Geometry: final body of the model. Coordinates: model frame, mm. A direction names the side the tool comes from. Give positions to 0.01 mm unless a question says otherwise; leave off trailing zeros. Write each loop counter-clockwise with the first axis right and the second up, starting at its lowest first coordinate (ties: lowest second). Pieces come first, ordered by that corner, then holes.
Q1. Mould query, pull axis X, two halves, no side actions, for faces 3 (the cylindrical face through (19.14, -19.1, 0.28)), 4 (the cylindrical face through (-19.1, -19.14, 0.28)), 5 (the cylindrical face through (-17, -16.5, 0)), 6 (the cylindrical face through (12.5, 15.1, 0)). Classes: +X half, -X half, draft (parallel to the pull), parting line (faces both ways), or undercut.
Q2. Line query: line 1 (Y direction, x = -15, z = 1.2); line 2 (Y direction, x = 13, z = 0); line 3 (Z direction, x = 12.5, y = -12). Output: solid intervals per line, ascending.
Q3. Section D-D (y = 0). Return the cut outline in (x, z).
Q4. Section A-A (z = 1.5). Return the cut outline in (x, y), plus the area to 3 significant figures.
Q5. Section B-B (x = 15). Return the cut outline in (y, z), plus the area to 3 significant figures.
Q6. Pin query (flat end, axial travel): pin 1 Ø6.5 at (x, y) = (-15, -15) entering from -Z; pin 2 Ø4 at (x, z) = (3.5, 5.5) entering from -Y; pin 3 Ø1 at (x, z) = (0, 4) entering from -Y; pin 4 Ø4 at (x, y) = (15, 15) entering from -Z. Return the tip coordinate at first contact, or that it passes through.
Q7. Reachability of faces 1 (the flat face through (0, 0, -2.5)), 2 (the flat face through (-9, 14, 2.5)) from +Z, -Z, +X, -X, +Y, -Y: full face, straight path, thin tool, end or side. Return the list, or none.
from build123d import *

# Parameters (mm, degrees)
SKETCH1_W           = 40
SKETCH1_H           = 40
SKETCH1_R           = 2.5
SKETCH1_R_2         = 16
BOSS_EXTRUDE1_DEPTH = 2.5
BOSS_EXTRUDE2_START = 2.5
SKETCH1_5_R         = 16
BOSS_EXTRUDE2_DEPTH = 6
FILLET1_R           = 0.5
FILLET2_R           = 3


with BuildPart() as part:
    # Sketch1 → Boss-Extrude1 (new, symmetric)
    # profile 1 of 2: a face of its own
    with BuildSketch(Plane.XY):
        Rectangle(SKETCH1_W, SKETCH1_H)
        with Locations((-15, -15)):
            Circle(SKETCH1_R, mode=Mode.SUBTRACT)
        with Locations((15, -15)):
            Circle(SKETCH1_R, mode=Mode.SUBTRACT)
        with Locations((15, 15)):
            Circle(SKETCH1_R, mode=Mode.SUBTRACT)
        with Locations((-15, 15)):
            Circle(SKETCH1_R, mode=Mode.SUBTRACT)
        Circle(SKETCH1_R_2, mode=Mode.SUBTRACT)
    # profile 2 of 2: a face of its own
    with BuildSketch(Plane.XY):
        Circle(SKETCH1_R_2)
    extrude(amount=BOSS_EXTRUDE1_DEPTH, both=True)

    # Sketch1<5> → Boss-Extrude2 (add)
    with BuildSketch(Plane.XY.offset(BOSS_EXTRUDE2_START)):
        Circle(SKETCH1_5_R)
    extrude(amount=BOSS_EXTRUDE2_DEPTH)

    # Fillet1
    fillet1_edges = [part.edges().sort_by_distance(p)[0] for p in [
        (0, -20, -2.5),
        (-20, 0, -2.5),
        (0, 20, -2.5),
        (20, 0, -2.5),
    ]]
    fillet(fillet1_edges, radius=FILLET1_R)

    # Fillet2
    # the kernel refuses this fillet: 3 mm, written as the material it takes off along each edge
    with BuildSketch(Plane(origin=(-17, 17, -2.5), x_dir=(-1, 0, 0), z_dir=(0, -1, 0))) as fillet2_piece_1:
        with BuildLine():
            CenterArc((2.5, -0.5), 0.5, 0, 90)
            Line((3, -0.5), (3, 0))
            Line((3, 0), (2.5, 0))
        make_face()
    revolve(axis=Axis((-17, 17, -2.5), (0, 0, -1)), revolution_arc=90, mode=Mode.SUBTRACT)
    with BuildSketch(Plane(origin=(-17, -17, -2.5), x_dir=(0, -1, 0), z_dir=(1, 0, 0))) as fillet2_piece_2:
        with BuildLine():
            CenterArc((2.5, -0.5), 0.5, 0, 90)
            Line((3, -0.5), (3, 0))
            Line((3, 0), (2.5, 0))
        make_face()
    revolve(axis=Axis((-17, -17, -2.5), (0, 0, -1)), revolution_arc=90, mode=Mode.SUBTRACT)
    with BuildSketch(Plane(origin=(17, 17, -2.5), x_dir=(0, 1, 0), z_dir=(-1, 0, 0))) as fillet2_piece_3:
        with BuildLine():
            CenterArc((2.5, -0.5), 0.5, 0, 90)
            Line((3, -0.5), (3, 0))
            Line((3, 0), (2.5, 0))
        make_face()
    revolve(axis=Axis((17, 17, -2.5), (0, 0, -1)), revolution_arc=90, mode=Mode.SUBTRACT)
    with BuildSketch(Plane(origin=(17, -17, -2.5), x_dir=(1, 0, 0), z_dir=(0, 1, 0))) as fillet2_piece_4:
        with BuildLine():
            CenterArc((2.5, -0.5), 0.5, 0, 90)
            Line((3, -0.5), (3, 0))
            Line((3, 0), (2.5, 0))
        make_face()
    revolve(axis=Axis((17, -17, -2.5), (0, 0, -1)), revolution_arc=90, mode=Mode.SUBTRACT)
    with BuildSketch(Plane(origin=(20, -20, 10), x_dir=(0, 1, 0), z_dir=(0, 0, -1)), Plane(origin=(-20, -20, 10), x_dir=(1, 0, 0), z_dir=(0, 0, -1)), Plane(origin=(-20, 20, -2.5), x_dir=(1, 0, 0), z_dir=(0, 0, 1)), Plane(origin=(20, 20, -2.5), x_dir=(0, -1, 0), z_dir=(0, 0, 1))) as fillet2_piece_5:
        with BuildLine():
            CenterArc((FILLET2_R, -FILLET2_R), FILLET2_R, 90, 90)
            Line((0, -FILLET2_R), (0, 0))
            Line((0, 0), (FILLET2_R, 0))
        make_face()
    extrude(amount=12.5, mode=Mode.SUBTRACT)


solid = part.part
Computed:
1. face 3: +X half
1. face 4: -X half
1. face 5: undercut
1. face 6: undercut
2. line 1: y = -20 to -17.5, -12.5 to 12.5, 17.5 to 20
2. line 2: y = -20 to -16.5, -13.5 to 13.5, 16.5 to 20
2. line 3: z = -2.5 to 2.5
3. outline: (-20, -2) arc R0.5 ccw to (-19.5, -2.5) - (19.5, -2.5) arc R0.5 ccw to (20, -2) - (20, 2.5) - (16, 2.5) - (16, 8.5) - (-16, 8.5) - (-16, 2.5) - (-20, 2.5) - close
4. outline: (-20, -17) arc R3 ccw to (-17, -20) - (17, -20) arc R3 ccw to (20, -17) - (20, 17) arc R3 ccw to (17, 20) - (-17, 20) arc R3 ccw to (-20, 17) - close; hole circle Ø5 at (-15, -15); hole circle Ø5 at (-15, 15); hole circle Ø5 at (15, -15); hole circle Ø5 at (15, 15)
4. area: 1,510 mm2
5. outline: (-20, -2) arc R0.5 ccw to (-19.5, -2.5) - (-17.5, -2.5) - (-17.5, 2.5) - (-20, 2.5) - close; (-12.5, -2.5) - (12.5, -2.5) - (12.5, 2.5) - (5.57, 2.5) - (5.57, 8.5) - (-5.57, 8.5) - (-5.57, 2.5) - (-12.5, 2.5) - close; (17.5, -2.5) - (19.5, -2.5) arc R0.5 ccw to (20, -2) - (20, 2.5) - (17.5, 2.5) - close
5. area: 217 mm2
6. pin 1: stops at z = -2.5
6. pin 2: stops at y = -15.93
6. pin 3: stops at y = -16
6. pin 4: passes through
7. face 1: -Z, +X, -X, +Y, -Y
7. face 2: +Z
